The listing builds one solid part. Answer for the finished solid, in the listing's coordinates (mm). A direction names the side the tool comes from. Give positions to 0.01 mm unless a question says otherwise; leave off trailing zeros. Order: outer loops, then holes, each group sorted by start corner. A loop starts at its lowest first (then second) coordinate and runs counter-clockwise, first axis right, second up. Notation, with made-up numbers: (59, 60.5) - (91, 60.5) arc R27 ccw to (91, 91.5) - close; hole circle Ø3 at (-15.5, 23.5). An arc over 180 degrees is marked (long way). Use CSV: the item, a comma, the result in double quotes.
```python
from build123d import *

# Parameters (mm, degrees)
SKETCH1_R               = 10
BOSS_EXTRUDE1_DEPTH     = 95
SKETCH4_W               = 10
SKETCH4_H               = 15
BOSS_EXTRUDE3_DEPTH     = 15
SKETCH5_R               = 5
CUT_EXTRUDE2_DEPTH      = 15
FILLET1_R               = 5
SKETCH9_R               = 10
BOSS_EXTRUDE4_DEPTH     = 20
SKETCH10_W              = 10
SKETCH10_H              = 36.273756528
CUT_EXTRUDE4_DEPTH      = 20
SKETCH12_R              = 5
CUT_EXTRUDE5_DEPTH      = 11
CUT_EXTRUDE5_DEPTH_BACK = 11


with BuildPart() as part:
    # Sketch1 → Boss-Extrude1 (new body)
    with BuildSketch(Plane(origin=(0, 0, 0), x_dir=(1, 0, 0), z_dir=(0, 1, 0))):
        Circle(SKETCH1_R)
    extrude(amount=BOSS_EXTRUDE1_DEPTH)

    # Sketch4 → Boss-Extrude3 (add)
    with BuildSketch(Plane.XZ):
        Rectangle(SKETCH4_W, SKETCH4_H)
    extrude(amount=BOSS_EXTRUDE3_DEPTH)

    # Sketch5 → Cut-Extrude2 (cut)
    with BuildSketch(Plane.ZY.offset(5)):
        with Locations((0, -7.5)):
            Circle(SKETCH5_R)
    extrude(amount=-CUT_EXTRUDE2_DEPTH, mode=Mode.SUBTRACT)

    # Fillet1
    fillet1_edges = [part.edges().sort_by_distance(p)[0] for p in [
        (0, -15, -7.5),
        (0, -15, 7.5),
    ]]
    fillet(fillet1_edges, radius=FILLET1_R)

    # Sketch9 → Boss-Extrude4 (add)
    with BuildSketch(Plane(origin=(0, 95, 0), x_dir=(1, 0, 0), z_dir=(0, 1, 0))):
        Circle(SKETCH9_R)
    extrude(amount=BOSS_EXTRUDE4_DEPTH)

    # Sketch10 → Cut-Extrude4 (cut)
    with BuildSketch(Plane(origin=(0, 115, 0), x_dir=(1, 0, 0), z_dir=(0, 1, 0))):
        Rectangle(SKETCH10_W, SKETCH10_H)
    extrude(amount=-CUT_EXTRUDE4_DEPTH, mode=Mode.SUBTRACT)

    # Sketch12 → Cut-Extrude5 (cut, two sides)
    with BuildSketch(Plane(origin=(0, 0, 0), x_dir=(0, 0, -1), z_dir=(1, 0, 0))) as cut_extrude5_sk:
        with Locations((0, 105)):
            Circle(SKETCH12_R)
    extrude(amount=CUT_EXTRUDE5_DEPTH, mode=Mode.SUBTRACT)
    extrude(cut_extrude5_sk.sketch, amount=-CUT_EXTRUDE5_DEPTH_BACK, mode=Mode.SUBTRACT)


solid = part.part
```
Item 1: Which of the six approach directions +Z, -Z, +X, -X, +Y, -Y give full straight-line access (tool end or side, diameter ignored) to faces 1 (the face through (0, -5, -7.5)), 2 (the face through (-5, 110, 2)), 3 (the face through (0, -5, 7.5)), 4 (the face through (-5, -2, 0))?
Taken from the geometry:
face 1,"-Z, +X, -X, -Y"
face 2,"+Z, -Z, +Y"
face 3,"+Z, +X, -X, -Y"
face 4,"+Z, -Z, -X, -Y"
Item 2: The mould has two halves that part along Z. Classify faces 5 (the face through (7, 102, 4)), 6 (the face through (0.07, -13.5, -6.07)), 7 (the face through (-7, 102, 4)), 8 (the face through (0, -15, 0)): +Z half, -Z half, draft (parallel to the pull), parting line (faces both ways), or undercut.
Taken from the geometry:
face 5,"undercut"
face 6,"-Z half"
face 7,"undercut"
face 8,"draft"
Item 3: The part is cut by section B-B (z = 0). Give the vertices of the cut face in (x, y).
Taken from the geometry:
outline,"(-10, 0) - (-5, 0) - (-5, -2.5) - (5, -2.5) - (5, 0) - (10, 0) - (10, 100) - (5, 100) - (5, 95) - (-5, 95) - (-5, 100) - (-10, 100) - close; (-10, 110) - (-5, 110) - (-5, 115) - (-10, 115) - close; (-5, -15) - (5, -15) - (5, -12.5) - (-5, -12.5) - close; (5, 110) - (10, 110) - (10, 115) - (5, 115) - close"
Item 4: Find the intervals of material crossed by line 1 along Y through (x, z) = (1.75, 0); line 2 along Y through (x, z) = (-8.85, 0); line 3 along Z through (x, y) = (7.35, 105), in increasing order.
Taken from the geometry:
line 1,"-15 to -12.5, -2.5 to 95"
line 2,"0 to 100, 110 to 115"
line 3,"-6.78 to -5, 5 to 6.78"
Item 5: Each of these flat-tipped pins is pushed along its axis until it touches: pin 1 (4.5 mm diameter, centred on y = -10.5, z = -2, fed in from -X); pin 2 (5 mm diameter, centred on y = 108, z = 4, fed in from -X); pin 3 (1 mm diameter, centred on y = 97, z = 2, fed in from -X). Where does it stop, or does it pass through?
Taken from the geometry:
pin 1,"x = -5"
pin 2,"x = -9.79"
pin 3,"x = -9.89"
Item 6: The part is cut by section C-C (y = 105). Give the vertices of the cut face in (x, z), and give its area (3 significant figures).
Taken from the geometry:
outline,"(-8.66, -5) arc R10 ccw to (-5, -8.66) - (-5, -5) - close; (-8.66, 5) - (-5, 5) - (-5, 8.66) arc R10 ccw to start; (5, -8.66) arc R10 ccw to (8.66, -5) - (5, -5) - close; (5, 5) - (8.66, 5) arc R10 ccw to (5, 8.66) - close"
area,"31.5 mm^2"
Item 7: The part is cut by section A-A (y = -7.5). Give the vertices of the cut face in (x, z), and give its area (3 significant figures).
Taken from the geometry:
outline,"(-5, -7.5) - (5, -7.5) - (5, -5) - (-5, -5) - close; (-5, 5) - (5, 5) - (5, 7.5) - (-5, 7.5) - close"
area,"50.0 mm^2"
Item 8: The part is cut by section D-D (x = -2). Give the vertices of the cut face in (y, z).
Taken from the geometry:
outline,"(-15, -2.5) arc R5 ccw to (-10, -7.5) - (0, -7.5) - (0, -9.8) - (95, -9.8) - (95, 9.8) - (0, 9.8) - (0, 7.5) - (-10, 7.5) arc R5 ccw to (-15, 2.5) - close; hole circle Ø10 at (-7.5, 0)"
